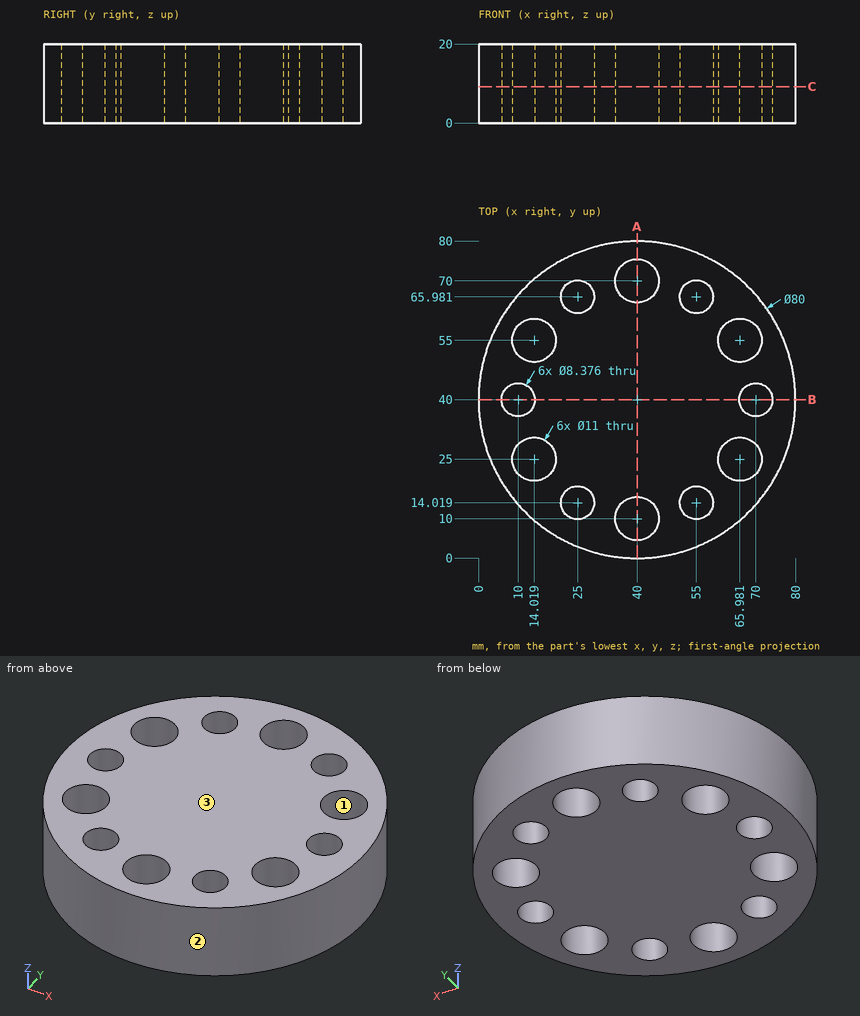
Study the drawing (mm; zero at the part's minimum x, y, z) and answer. Coordinates: 2 decimals unless noted, no trailing zeros. Loops run counter-clockwise (first coordinate to the right, second up) from the corner with the lowest first, then second, coordinate; pieces in that order, holes last. Notation, with made-up numbers: M 65,35.25 L 72,35.25 A16 ccw 72,49.25 Z; hole C 40.5,81.5 d11. An arc over 180 degrees is marked long. Answer in a Markdown table with one row per item. Add a question column.
1. Find section C-C, the plane z = 9.25. State how many separate pieces and enclosed holes the cut face has, then the cut area to 3 significant figures.
2. Find section A-A, the plane x = 40. Write down the section's boundary in (y, z).
3. The mould has two halves that part along Y. Classify the marked faces 1, 2 and 3: pulls with the +Y half, pulls with the -Y half, needs draft (parallel to the pull), parting line crosses it, or undercut.
4. Flat-ended cylindrical pins translate along their axes: P1, Ø10, axis at y = 71, z = 14, coming from the -X side; P2, Ø13.5, axis at x = 10, y = 40, coming from the -Z side; P3, Ø5, axis at y = 45.5, z = 11, coming from the +X side; P4, Ø5, axis at y = 51.5, z = 10, coming from the +X side. Find the tip coordinate at first contact, or state that the pin passes through.
5. Find section B-B, the plane y = 40. Write down the section's boundary in (x, z).
6. Consider L1, parallel to Y at x = 39.5, z = 8.75; L2, parallel to X at y = 55, z = 14.75; L3, parallel to Y at x = 17, z = 3.5 (1 decimal). Determine where each line is inside the solid, lowest interval first.
Reported:
| question | item | result |
|---|---|---|
| 1 | separate pieces | 1 |
| 1 | enclosed holes | 12 |
| 1 | area | 4,130 mm^2 |
| 2 | outline | M 0,0 L 4.5,0 L 4.5,20 L 0,20 Z; M 15.5,0 L 64.5,0 L 64.5,20 L 15.5,20 Z; M 75.5,0 L 80,0 L 80,20 L 75.5,20 Z |
| 3 | face 1 | undercut |
| 3 | face 2 | parting line crosses it |
| 3 | face 3 | needs draft |
| 4 | P1 | stops at x = 9.6 |
| 4 | P2 | stops at z = 0 |
| 4 | P3 | stops at x = 79.89 |
| 4 | P4 | stops at x = 78.97 |
| 5 | outline | M 0,0 L 5.81,0 L 5.81,20 L 0,20 Z; M 14.19,0 L 65.81,0 L 65.81,20 L 14.19,20 Z; M 74.19,0 L 80,0 L 80,20 L 74.19,20 Z |
| 6 | L1 | y = 0 to 4.52, 15.48 to 64.52, 75.48 to 80 |
| 6 | L2 | x = 2.92 to 8.52, 19.52 to 60.48, 71.48 to 77.08 |
| 6 | L3 | y = 7.3 to 20.4, 29.6 to 50.4, 59.6 to 72.7 |
